Design review of the part shown in the three views and the two pictorial views. Dimensions are in mm from the part's minimum x, y and z. A direction names the side the tool comes from. Give positions to 0.01 mm unless a question says otherwise; leave off trailing zeros. Loops run counter-clockwise (first coordinate to the right, second up) from the corner with the lowest first, then second, coordinate; pieces in that order, holes last. Notation, with made-up numbers: (2.5, -4.5) - (50.5, -4.5) arc R23 cw to (50.5, 23.5) - close; hole circle Ø7 at (-15, 62). An arc over 180 degrees is marked (long way). Answer as a JSON object with one key per item and string values.
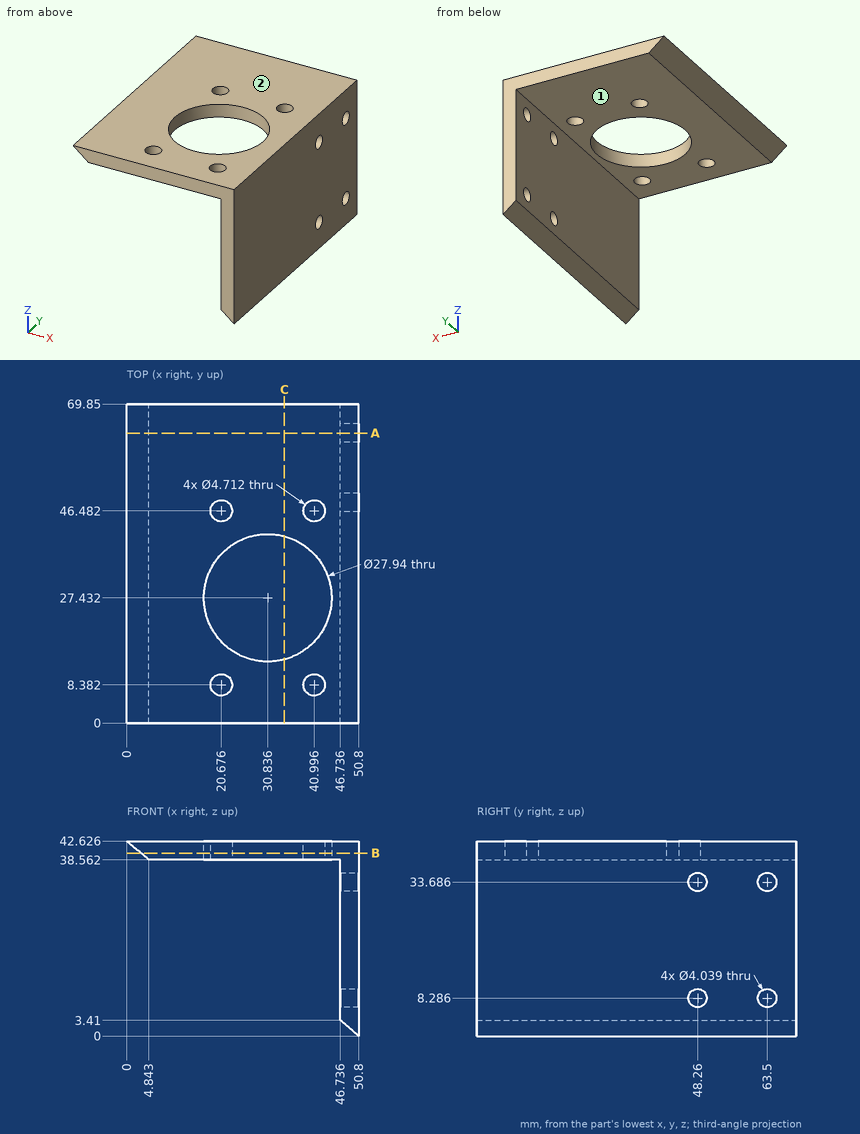
Q1. For the marked faces 1 and 2, list the 3-axis set-ups (+Z, -Z, +X, -X, +Y, -Y) from which the entire face can be reached by the end or side of a thin tool; tool diameter is ignored.
Results:
{"face 1": "-Z, -X, +Y, -Y", "face 2": "+Z, +X, -X, +Y, -Y"}
Q2. Consider section B-B, the plane z = 40. State how many separate pieces and enclosed holes the cut face has, plus the area to 3 significant figures.
Results:
{"separate pieces": "1", "enclosed holes": "5", "area": "2,650 mm^2"}
Q3. Consider section C-C, the plane x = 34.5. State the section outline as (y, z) points, plus the area to 3 significant figures.
Results:
{"outline": "(0, 38.56) - (13.95, 38.56) - (13.95, 42.63) - (0, 42.63) - close; (40.91, 38.56) - (69.85, 38.56) - (69.85, 42.63) - (40.91, 42.63) - close", "area": "174 mm^2"}
Q4. Consider section A-A, the plane y = 63.5. State the section outline as (x, z) points (1 decimal).
Results:
{"outline": "(0, 42.6) - (4.8, 38.6) - (46.7, 38.6) - (46.7, 35.7) - (50.8, 35.7) - (50.8, 42.6) - close; (46.7, 3.4) - (50.8, 0) - (50.8, 6.3) - (46.7, 6.3) - close; (46.7, 10.3) - (50.8, 10.3) - (50.8, 31.7) - (46.7, 31.7) - close"}
Q5. Clearance check with flat-ended pins moving along their axes: pin 1 Ø6 at (y, z) = (20.5, 25.5) entering from -X; pin 2 Ø6 at (x, y) = (20.68, 8.38) entering from -Z. State where each tip first meets the part, or that it passes through.
Results:
{"pin 1": "stops at x = 46.74", "pin 2": "stops at z = 38.56"}
Q6. To check wall thickness, follow probe 1 along X at (y, z) = (67, 20.5); probe 2 along Z at (x, y) = (14.5, 41); probe 3 along Z at (x, y) = (3, 9) (1 decimal). State the ranges of each line that lie inside material, in increasing order. Write a range as [from, to].
Results:
{"probe 1": "x = [46.74, 50.8]", "probe 2": "z = [38.56, 42.63]", "probe 3": "z = [40.1, 42.6]"}
